Geometry check sheet. Reference: the model listing, model coordinates, mm. A direction names the side the tool comes from. Give positions to 0.01 mm unless a question says otherwise; leave off trailing zeros. Loops run counter-clockwise (first coordinate to the right, second up) from the corner with the lowest first, then second, coordinate; pieces in that order, holes last. Notation, with made-up numbers: (-28, 76.5) -> (30, 76.5) arc R8 ccw to (30, 80.5) -> close; hole circle Ø4 at (6, 77). An arc over 180 degrees is marked (long way). One line per item, written item: value. Start each with the question number.
(1) Sectioned sample at B-B, the plane x = 0. Record the cut outline in (y, z).
(2) Draft check along Z on faces 4 (the face through (-5, -398, 1219.2)), 5 (the face through (-247.786, -337.342, 1294.333)), 6 (the face through (-6.11, -389.81, 26.29)). Enter one of: pulls with the +Z half, pulls with the -Z half, needs draft (parallel to the pull), parting line crosses it, or undercut.
(3) Tool access check on faces 1 (the face through (246.36, -339.71, 1294.33)), 2 (the face through (3, -390, 276.248)), 3 (the face through (-49.599, 377.758, 676.199)). Record the directions out of +Z, -Z, +X, -X, +Y, -Y that give a thin tool (end or side, any length) a straight path to the whole face; none if there is none.
(4) Sectioned sample at D-D, the plane x = 297. Record the cut outline in (y, z), then the cut area to 3 significant figures.
(5) Sectioned sample at A-A, the plane y = 0. Record the cut outline in (x, z).
(6) Gauge pin test, flat ends, axial feed: pin 1 Ø3 at (x, y) = (-259.5, -176) entering from +Z; pin 2 Ø3 at (y, z) = (-57, 225) entering from +X; pin 3 Ø10 at (y, z) = (93.5, 499.5) entering from +X. Record the tip position at first contact, or that the pin passes through.
(7) Sectioned sample at C-C, the plane z = 508.5. Record the cut outline in (x, y).
(8) Scan lines: line 1 along Y through (x, z) = (0, 758); line 2 along X through (y, z) = (49.5, 37). Record each from-to range of solid material in increasing order. Write a range as from..to.
from build123d import *

# Parameters (mm, degrees)
F0_R     = 457.2
F0_R_2   = 381
F1_DEPTH = 1371.6
F5_DEPTH = 457.2
F7_START = 1219.2
F7_DEPTH = 152.4


with BuildPart() as f1:
    # F0 (on Top) → F1 (new body)
    with BuildSketch(Plane.XY):
        Circle(F0_R)
        Circle(F0_R_2, mode=Mode.SUBTRACT)
    extrude(amount=F1_DEPTH)

    # F2 (on Right) → F3 (revolve)
    with BuildSketch(Plane.YZ):
        with BuildLine():
            ThreePointArc((0, -381), (-269.4076836321, -269.4076836321), (-381, 0))
            Line((-381, 0), (-457.2, 0))
            ThreePointArc((-457.2, 0), (-323.2892203585, -323.2892203585), (0, -457.2))
            Line((0, -457.2), (0, -381))
        make_face()
    revolve(axis=Axis((0, 0, -419.1), (0, 0, 1)))

    # F4 (on Front) → F5 (cut)
    with BuildSketch(Plane.XZ):
        with BuildLine():
            ThreePointArc((-250.6338357925, 276.2475907803), (-0.6155371666, 26.2292921543), (249.4027614594, 276.2475907803))
            Line((249.4027614594, 276.2475907803), (-250.6338357925, 276.2475907803))
        make_face()
    extrude(amount=F5_DEPTH, mode=Mode.SUBTRACT)

    # F6 (on Top) → F7 (cut)
    with BuildSketch(Plane.XY.offset(F7_START)):
        with BuildLine():
            Line((268.4118130728, -370.1174659523), (0, 0))
            Line((0, 0), (-270.6568666844, -368.4789010467))
            ThreePointArc((-270.6568666844, -368.4789010467), (-1.3897086627, -457.1978879105), (268.4118130728, -370.1174659523))
        make_face()
    extrude(amount=F7_DEPTH, mode=Mode.SUBTRACT)


solid = f1.part
Calculated:
1. outline: (-457.2, 0) arc R457.2 ccw to (457.2, 0) -> (457.2, 1371.6) -> (381, 1371.6) -> (381, 0) arc R381 cw to (-381, 0) -> (-381, 26.23) -> (-457.2, 26.23) -> close; (-457.2, 276.25) -> (-381, 276.25) -> (-381, 1219.2) -> (-457.2, 1219.2) -> close
2. face 4: pulls with the +Z half
2. face 5: needs draft
2. face 6: undercut
3. face 1: +Z, -Y
3. face 2: -Y
3. face 3: +Z
4. outline: (-347.6, 0) arc R347.6 ccw to (347.6, 0) -> (347.6, 1371.6) -> (238.65, 1371.6) -> (238.65, 0) arc R238.65 cw to (-238.65, 0) -> (-238.65, 1371.6) -> (-347.6, 1371.6) -> close
4. area: 399,000 mm2
5. outline: (-457.2, 0) arc R457.2 ccw to (457.2, 0) -> (457.2, 1371.6) -> (381, 1371.6) -> (381, 0) arc R381 cw to (-381, 0) -> (-381, 1371.6) -> (-457.2, 1371.6) -> close
6. pin 1: stops at z = -214.25
6. pin 2: stops at x = 453.82
6. pin 3: stops at x = 448.55
7. outline: circle Ø914.4 at (0, 0); hole circle Ø762 at (0, 0)
8. line 1: y = -457.2..-381, 381..457.2
8. line 2: x = -454.51..-377.77, 377.77..454.51
